Design review of the part shown in the three views and the two pictorial views. Dimensions are in mm from the part's minimum x, y and z. A direction names the side the tool comes from. Give positions to 0.01 mm unless a question says otherwise; leave off trailing zeros. Loops run counter-clockwise (first coordinate to the right, second up) from the corner with the lowest first, then second, coordinate; pieces in that order, holes last. Notation, with made-up numbers: (-33, 24) - (-25, 24) arc R14 cw to (-25, 48) - close; hole circle Ø10 at (52.25, 58.5). An arc over 180 degrees is marked (long way). Answer in a Markdown table with one row per item.
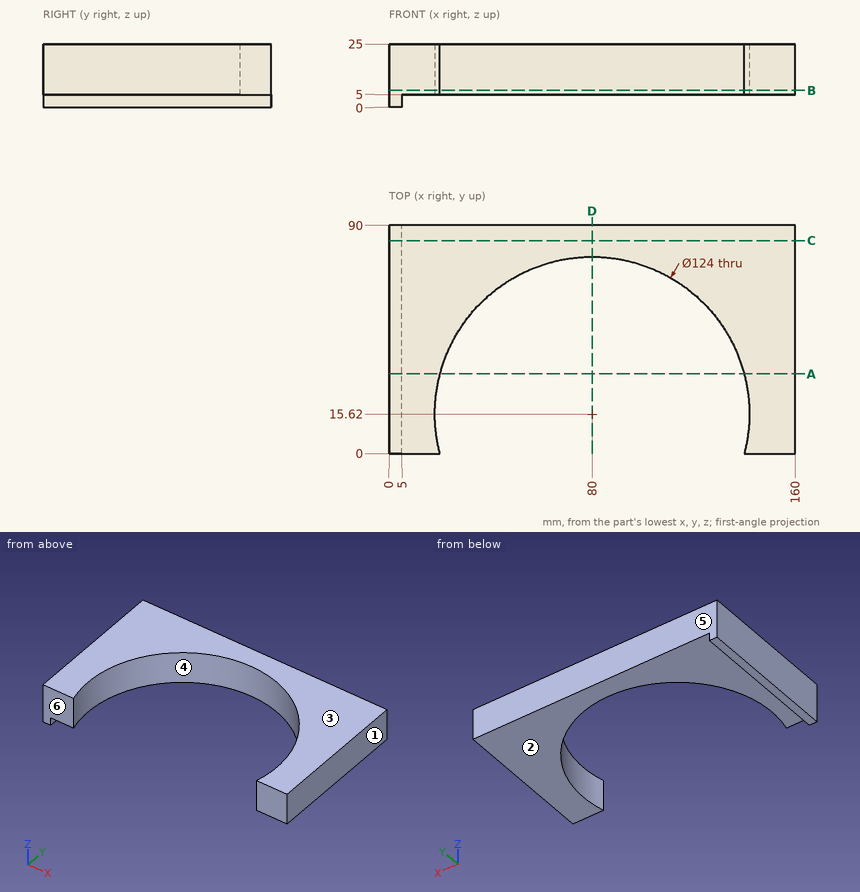
1. Wall thickness on line 1 (X direction, y = 61.5, z = 4.25); line 2 (X direction, y = 64, z = 18.5) (1 decimal); line 3 (Z direction, x = 10.5, y = 53): over which ranges is each line inside the solid? List them lowest first. Write a range as [from, to].
Values:
| item | result |
|---|---|
| line 1 | x = [0, 5] |
| line 2 | x = [0, 41.2], [118.8, 160] |
| line 3 | z = [5, 25] |
2. Clearance check with flat-ended pins moving along their axes: pin 1 (2.5 mm diameter, centred on y = 66.5, z = 1.5, fed in from +X); pin 2 (5 mm diameter, centred on y = 10, z = 17, fed in from -X); pin 3 (3 mm diameter, centred on x = 125.5, z = 13.5, fed in from -Y) (1 decimal). State where each tip first meets the part, or that it passes through.
Values:
| item | result |
|---|---|
| pin 1 | stops at x = 5 |
| pin 2 | stops at x = 0 |
| pin 3 | stops at y = 56.1 |
3. For the marked faces 1 and 2, list the 3-axis set-ups (+Z, -Z, +X, -X, +Y, -Y) from which the entire face can be reached by the end or side of a thin tool; tool diameter is ignored.
Values:
| item | result |
|---|---|
| face 1 | +Z, -Z, +X, +Y, -Y |
| face 2 | -Z, +X, +Y, -Y |
4. We need section B-B, the plane z = 6.75. Give the boundary of the cut face in (x, y).
Values:
| item | result |
|---|---|
| outline | (0, 0) - (20, 0) arc R62 cw (long way) to (140, 0) - (160, 0) - (160, 90) - (0, 90) - close |
5. We need section A-A, the plane y = 31.5. Give the boundary of the cut face in (x, z), and give its area (3 significant figures).
Values:
| item | result |
|---|---|
| outline | (0, 0) - (5, 0) - (5, 5) - (20.07, 5) - (20.07, 25) - (0, 25) - close; (139.93, 5) - (160, 5) - (160, 25) - (139.93, 25) - close |
| area | 828 mm^2 |
6. We need section C-C, the plane y = 84. Give the boundary of the cut face in (x, z), and give its area (4 significant figures).
Values:
| item | result |
|---|---|
| outline | (0, 0) - (5, 0) - (5, 5) - (160, 5) - (160, 25) - (0, 25) - close |
| area | 3,225 mm^2 |
7. We need section D-D, the plane x = 80. Give the boundary of the cut face in (y, z), and give its area (3 significant figures).
Values:
| item | result |
|---|---|
| outline | (77.62, 5) - (90, 5) - (90, 25) - (77.62, 25) - close |
| area | 248 mm^2 |
8. Mouldability with a two-part tool opening along Y and no side actions: class the marked faces 3, 4, 5 and 6 as released by +Y, released by -Y, zero draft, split by the parting line, or undercut.
Values:
| item | result |
|---|---|
| face 3 | zero draft |
| face 4 | undercut |
| face 5 | released by +Y |
| face 6 | released by -Y |
